For this review, take the finished solid that the model builds, in its own axes (mm). Round coordinates to 2 decimals unless told otherwise and drop trailing zeros. Order: outer loops, then holes, each group sorted by start corner. A loop starts at its lowest first (then second) coordinate and runs counter-clockwise, first axis right, second up. Notation, with made-up numbers: (63, 43) - (82, 43) arc R27 cw to (82, 82) - close; hole circle Ø2 at (-29.5, 20). An arc over 180 degrees is marked (long way). Write each question's results on one line, items separated by ' | '. Start each with the question number.
(1) Take a section at C-C, the plane x = -2.75. Give the boundary of the cut face in (y, z), plus the area to 3 significant figures.
(2) Insertion check: pin 1 Ø1.5 at (x, y) = (6.43, -6.64) entering from -Z. The pin has a flat end and moves straight along its axis. Give the tip position at first contact, or say it passes through.
(3) Take a section at B-B, the plane z = 0.8. Give the number of separate pieces and of enclosed holes in the cut face, plus the area to 3 significant figures.
(4) Draft analysis for pull direction X (two halves, no side actions). For faces 1 (the cylindrical face through (-10.116, -5.782, 0.805)), 2 (the cylindrical face through (10.8, -8.2, 0.8)), 3 (the cylindrical face through (-5.418, -7.163, 0.805)), 4 (the flat face through (0, 0, 0)), state which applies: pulls with the +X half, pulls with the -X half, needs draft (parallel to the pull), parting line crosses it, or undercut.
(5) For L1, parallel to Y at x = -9.18, z = 1.25; L2, parallel to X at y = 7.25, z = 1.25; L3, parallel to X at y = -6, z = 0.3, list the stretches that pass through material, from the lowest coordinate up. Write a range as from..to.
(6) Take a section at A-A, the plane x = 6.43. Give the boundary of the cut face in (y, z), plus the area to 3 significant figures.
```python
from build123d import *

# Parameters (mm, degrees)
BOSS_EXTRUDE1_DEPTH = 1.5875
SKETCH2_R           = 1.27
SKETCH2_R_2         = 0.5
CUT_EXTRUDE1_DEPTH  = 15.566988579


with BuildPart() as part:
    # Sketch1 → Boss-Extrude1 (new body)
    with BuildSketch(Plane.XY):
        with BuildLine():
            Line((9.18, -8.89), (-9.18, -8.89))
            ThreePointArc((-9.18, -8.89), (-10.770990258, -8.230990258), (-11.43, -6.64))
            Line((-11.43, -6.64), (-11.43, 6.64))
            ThreePointArc((-11.43, 6.64), (-10.770990258, 8.230990258), (-9.18, 8.89))
            Line((-9.18, 8.89), (9.18, 8.89))
            ThreePointArc((9.18, 8.89), (10.770990258, 8.230990258), (11.43, 6.64))
            Line((11.43, 6.64), (11.43, -6.64))
            ThreePointArc((11.43, -6.64), (10.770990258, -8.230990258), (9.18, -8.89))
        make_face()
    extrude(amount=BOSS_EXTRUDE1_DEPTH)

    # Sketch2 → Cut-Extrude1 (cut, through all)
    with BuildSketch(Plane.XY.offset(1.5875)):
        with Locations((-9.18, 6.64)):
            Circle(SKETCH2_R)
        with Locations((6.43, 6.64)):
            Circle(SKETCH2_R)
        with Locations((6.43, -6.64)):
            Circle(SKETCH2_R)
        with Locations((-9.18, -6.64)):
            Circle(SKETCH2_R)
        with Locations((-5.309559509, -6.675167708)):
            Circle(SKETCH2_R_2)
        with Locations((-2.769559509, -6.675167708)):
            Circle(SKETCH2_R_2)
        with Locations((-0.229559509, -6.675167708)):
            Circle(SKETCH2_R_2)
        with Locations((2.310440491, -6.675167708)):
            Circle(SKETCH2_R_2)
    extrude(amount=-CUT_EXTRUDE1_DEPTH, mode=Mode.SUBTRACT)


solid = part.part
```
Results below:
1) outline: (-8.89, 0) - (-7.17, 0) - (-7.17, 1.59) - (-8.89, 1.59) - close; (-6.18, 0) - (8.89, 0) - (8.89, 1.59) - (-6.18, 1.59) - close | area: 26.6 mm^2
2) pin 1: passes through
3) separate pieces: 1 | enclosed holes: 8 | area: 379 mm^2
4) face 1: undercut | face 2: pulls with the +X half | face 3: undercut | face 4: needs draft
5) L1: y = -8.89..-7.91, -5.37..5.37, 7.91..8.89 | L2: x = -11.35..-10.29, -8.07..5.32, 7.54..11.35 | L3: x = -11.43..-10.28, -8.08..5.33, 7.53..11.43
6) outline: (-8.89, 0) - (-7.91, 0) - (-7.91, 1.59) - (-8.89, 1.59) - close; (-5.37, 0) - (5.37, 0) - (5.37, 1.59) - (-5.37, 1.59) - close; (7.91, 0) - (8.89, 0) - (8.89, 1.59) - (7.91, 1.59) - close | area: 20.2 mm^2
